Can you work these out from the model? Positions are in its coordinate system, mm. Face numbers are marked on the shaded views. A direction names the side the tool comes from. Coordinates: 2 decimals unless noted, no trailing zeros. Order: outer loops, then holes, each group sorted by start corner. A loop starts at its lowest first (then second) coordinate and runs counter-clockwise, first axis right, second up. Notation, with made-up numbers: M 89,82.25 L 106,82.25 A16 ccw 106,99.25 Z; hole C 60,-3 d8. An arc over 180 degrees is marked long. Answer as a JSON object with one key per item and string values.
from build123d import *

# Parameters (mm, degrees)
SKETCH_3_W          = 80
SKETCH_3_H          = 55
EXTRUDE_2_DEPTH     = 55
SKETCH_4_W          = 40
SKETCH_4_H          = 40
CUT_EXTRUDE_2_DEPTH = 45
SKETCH_5_W          = 20
SKETCH_5_H          = 20
CUT_EXTRUDE_5_DEPTH = 15


with BuildPart() as part:
    # 草图3 → 凸台-拉伸2 (new body)
    with BuildSketch(Plane(origin=(0, 0, 0), x_dir=(1, 0, 0), z_dir=(0, 1, 0))):
        with Locations((40, 27.5)):
            Rectangle(SKETCH_3_W, SKETCH_3_H)
    extrude(amount=EXTRUDE_2_DEPTH)

    # 草图4 → 切除-拉伸2 (cut)
    with BuildSketch(Plane(origin=(80, 0, 0), x_dir=(0, 0, -1), z_dir=(1, 0, 0))):
        with Locations((35, 35)):
            Rectangle(SKETCH_4_W, SKETCH_4_H)
    extrude(amount=-CUT_EXTRUDE_2_DEPTH, mode=Mode.SUBTRACT)

    # 草图5 → 切除-拉伸5 (cut)
    with BuildSketch(Plane.ZY):
        with Locations((-45, 45)):
            Rectangle(SKETCH_5_W, SKETCH_5_H)
    extrude(amount=-CUT_EXTRUDE_5_DEPTH, mode=Mode.SUBTRACT)

    # loft from a face of the part (loft_11)
    loft([part.faces().sort_by_distance((35, 35, -35))[0], part.faces().sort_by_distance((15, 45, -45))[0]], mode=Mode.SUBTRACT)


solid = part.part
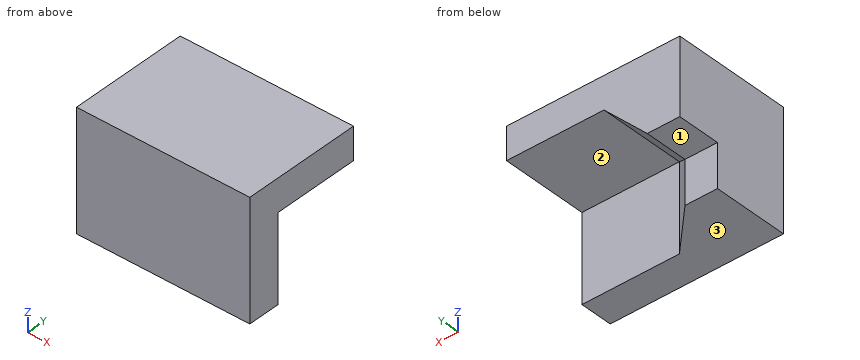
Item 1: Please list where these lines run through material, in increasing order: line 1 (Y direction, x = 37, z = -18.5); line 2 (Z direction, x = 72.5, y = 25); line 3 (Y direction, x = 11, z = -38).
Answers follow:
{"line 1": "y = 0 to 15", "line 2": "z = -15 to 0", "line 3": "y = 0 to 35"}
Item 2: I'm going to push flat-ended pins straight in: pin 1 (12 mm diameter, centred on x = 47.5, y = 43.5, fed in from -Z); pin 2 (12 mm diameter, centred on x = 38.5, y = 34.5, fed in from -Z); pin 3 (4.5 mm diameter, centred on x = 6, y = 44.5, fed in from -Z). Where does each tip first touch, or does it pass through?
Answers follow:
{"pin 1": "stops at z = -15", "pin 2": "stops at z = -17.5", "pin 3": "stops at z = -35"}
Item 3: Which directions (+Z, -Z, +X, -X, +Y, -Y) give clear straight access to the entire face, cutting with the end or side of a thin tool? Please do the marked faces 1, 2 and 3.
Answers follow:
{"face 1": "-Z, +X, -X, +Y", "face 2": "-Z, +X, +Y", "face 3": "-Z, +X, -X, +Y, -Y"}
Item 4: I want a section at A-A, the plane x = 68.5. Write out the boundary of the cut face in (y, z), plus the area to 4 significant figures.
Answers follow:
{"outline": "M 0,-55 L 15,-55 L 15,-15 L 55,-15 L 55,0 L 0,0 Z", "area": "1,425 mm^2"}
